from build123d import *

# Parameters (mm, degrees)
BOSS_EXTRUDE1_DEPTH = 144
BOSS_EXTRUDE2_DEPTH = 0.5
BOSS_EXTRUDE3_DEPTH = 0.5


with BuildPart() as part:
    # Sketch1 → Boss-Extrude1 (new body)
    with BuildSketch(Plane.XY):
        Polygon((-13, 2.5), (0, 0), (0, 33), (-13, 30.5), (-13.094423697, 30.991003223), (0.5, 33.605315473), (0.5, -0.605315473), (-13.094423697, 2.008996777), align=None)
    extrude(amount=BOSS_EXTRUDE1_DEPTH)

    # Sketch2 → Boss-Extrude2 (add)
    with BuildSketch(Plane(origin=(-6.214252513, 32.314113067, 0), x_dir=(0.9820064469806473, 0.18884739365012462, 0), z_dir=(-0.18884739365012462, 0.9820064469806473, 0))):
        with BuildLine():
            Line((-7.006238304, 0), (-7.006238304, 1.5))
            ThreePointArc((-7.006238304, 1.5), (-6.859791695, 1.853553391), (-6.506238304, 2))
            Line((-6.506238304, 2), (0.493761696, 2))
            ThreePointArc((0.493761696, 2), (0.847315086, 1.853553391), (0.993761696, 1.5))
            Line((0.993761696, 1.5), (0.993761696, 0))
            Line((0.993761696, 0), (-7.006238304, 0))
        make_face()
        with BuildLine():
            Line((-7.006238304, -144), (-7.006238304, -147.5))
            ThreePointArc((-7.006238304, -147.5), (-6.859791695, -147.853553391), (-6.506238304, -148))
            Line((-6.506238304, -148), (0.493761696, -148))
            ThreePointArc((0.493761696, -148), (0.847315086, -147.853553391), (0.993761696, -147.5))
            Line((0.993761696, -147.5), (0.993761696, -144))
            Line((0.993761696, -144), (-7.006238304, -144))
        make_face()
    extrude(amount=-BOSS_EXTRUDE2_DEPTH)

    # Sketch3 → Boss-Extrude3 (add)
    with BuildSketch(Plane(origin=(-0.094423697, -0.491003223, 0), x_dir=(0.9820064469806474, -0.18884739365012435, 0), z_dir=(-0.18884739365012435, -0.9820064469806474, 0))):
        with BuildLine():
            Line((-13.238202295, 147.5), (-13.238202295, 144))
            Line((-13.238202295, 144), (-5.238202295, 144))
            Line((-5.238202295, 144), (-5.238202295, 147.5))
            ThreePointArc((-5.238202295, 147.5), (-5.384648904, 147.853553391), (-5.738202295, 148))
            Line((-5.738202295, 148), (-12.738202295, 148))
            ThreePointArc((-12.738202295, 148), (-13.091755685, 147.853553391), (-13.238202295, 147.5))
        make_face()
        with BuildLine():
            Line((-5.238202295, 0), (-13.238202295, 0))
            Line((-13.238202295, 0), (-13.238202295, -1.5))
            ThreePointArc((-13.238202295, -1.5), (-13.091755685, -1.853553391), (-12.738202295, -2))
            Line((-12.738202295, -2), (-5.738202295, -2))
            ThreePointArc((-5.738202295, -2), (-5.384648904, -1.853553391), (-5.238202295, -1.5))
            Line((-5.238202295, -1.5), (-5.238202295, 0))
        make_face()
    extrude(amount=-BOSS_EXTRUDE3_DEPTH)


solid = part.part
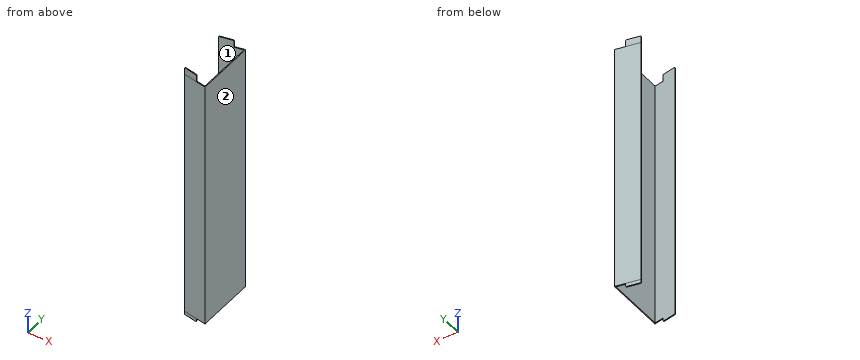
Model file for the job. Use its own axes, mm. Face numbers are marked on the shaded views. Coordinates: 2 decimals unless noted, no trailing zeros. Write each loop counter-clockwise with the first axis right and the second up, starting at its lowest first coordinate (ties: lowest second). Pieces come first, ordered by that corner, then holes. Notation, with made-up numbers: (30.5, 82) - (53.5, 82) arc R26 cw to (53.5, 102) - close; hole circle Ø1 at (-30.75, 75). An arc over 180 degrees is marked (long way). Write each question's results on one line, items separated by ' | '. Start each with the question number.
1) Cut at C-C (y = 5). Write the cut outline in (x, z), then the cut area to 3 significant figures.
2) Flat gauge pins, fed straight in: P1, Ø8, axis at x = -10, z = 41.5, coming from the +Y side; P2, Ø4, axis at y = 15.5, z = 61.5, coming from the -X side; P3, Ø2, axis at x = -6.5, z = 112.5, coming from the -Y side; P4, Ø3, axis at x = -3, y = 15.5, coming from the +Z side. Where does each tip first touch, or does it go through?
3) Probe line 1 along X through (y, z) = (16, 127); line 2 along Y through (x, z) = (-9.25, 17.5); line 3 along Y through (x, z) = (-4.75, 49.5). List the from-to ranges inside material, lowest first. Write a range as from..to.
4) Cut at B-B (z = 107). Write the cut outline in (x, y), then the cut area to 3 significant figures.
5) Cut at A-A (x = -3.5). Write the cut outline in (y, z).
6) Mould opens along X. For the marked faces 1 and 2 say: pulls with the +X half, pulls with the -X half, needs draft (parallel to the pull), parting line crosses it, or undercut.
Returned:
1) outline: (0, 0) - (0.5, 0) - (0.5, 144) - (0, 144) - close | area: 72.0 mm^2
2) P1: y = 32.36 | P2: x = 0 | P3: y = 0.55 | P4: through
3) line 1: 0..0.5 | line 2: 1.27..1.78, 31.22..31.73 | line 3: 0.4..0.91, 32.09..32.6
4) outline: (-13.09, 2.01) - (0.5, -0.61) - (0.5, 33.61) - (-13.09, 30.99) - (-13, 30.5) - (0, 33) - (0, 0) - (-13, 2.5) - close | area: 30.3 mm^2
5) outline: (0.16, 0) - (0.67, 0) - (0.67, 144) - (0.16, 144) - close; (32.33, 0) - (32.84, 0) - (32.84, 144) - (32.33, 144) - close
6) face 1: undercut | face 2: pulls with the +X half
